Design review of the part built by this model. Coordinates are the model's own, in mm. Face numbers are marked on the shaded views. Coordinates: 2 decimals unless noted, no trailing zeros. Loops run counter-clockwise (first coordinate to the right, second up) from the corner with the lowest first, then second, coordinate; pieces in that order, holes last.
Q1. Add section B-B on y = -2.5. Give the boundary of the cut face in (x, z), and give its area (3 significant figures).
Q2. For P1, Ø1.5, axis at y = -1, z = -9.5, coming from the +X side; P2, Ø3, axis at x = 0, z = 14, coming from the -Y side; P3, Ø8, axis at x = -2, y = -7, coming from the -Z side; P4, Ø1.5, axis at y = -5.5, z = -4.5, coming from the +X side, all flat-tipped, find the tip position at first contact; note any pin that passes through.
Q3. Add section C-C on z = -6. Give the boundary of the cut face in (x, y).
Q4. Wall thickness on probe 1 along Z at (x, y) = (0, 2.7); probe 2 along X at (y, z) = (-3.2, 0); probe 3 along X at (y, z) = (-1.75, 1): over which ranges is each line inside the solid? List them lowest first.
Q5. Draft analysis for pull direction X (two halves, no side actions). For the marked faces 1 and 2, state which applies: released by +X, released by -X, zero draft, split by the parting line, or undercut.
Q6. Add section D-D on x = 7.5. Give the boundary of the cut face in (y, z).
Q7. Add section A-A on y = 3.75. Give the boundary of the cut face in (x, z).
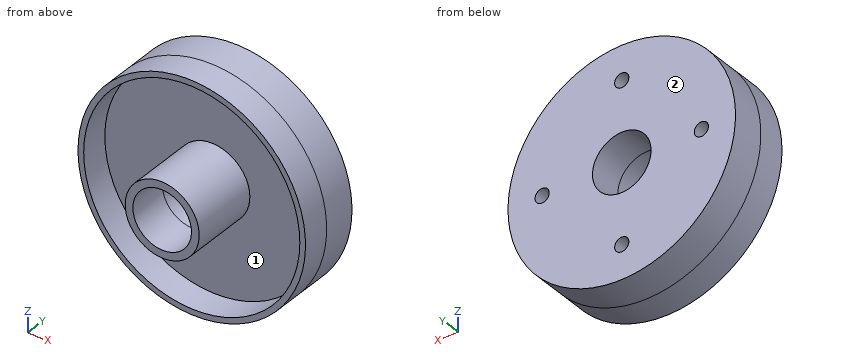
```python
from build123d import *

# Parameters (mm, degrees)
SKETCH_1_R             = 20
SKETCH_1_R_2           = 5.15
EXTRUDE_1_DEPTH        = 6
EXTRUDE_START          = 5
SKETCH_2_R             = 20
SKETCH_2_R_2           = 19
SKETCH_2_R_3           = 6.5
SKETCH_2_R_4           = 5.15
EXTRUDE_2_DEPTH        = 5
EXTRUDE_START_2        = 7
SKETCH_3_R             = 6.5
SKETCH_3_R_2           = 5.15
EXTRUDE_3_DEPTH        = 7
HOLE_WIZARD_M3_1_D     = 2.5
HOLE_WIZARD_M3_1_DEPTH = 5
HOLE_WIZARD_M3_1_TIP   = 0.751075774


with BuildPart() as part:
    # 草图1 → 凸台-拉伸1 (new body)
    with BuildSketch(Plane(origin=(0, 0, 0), x_dir=(1, 0, 0), z_dir=(0, 1, 0))):
        with Locations(Location((0, 0, 0), (0, 0, 270))):
            Circle(SKETCH_1_R)
        with Locations(Location((0, 0, 0), (0, 0, 270))):
            Circle(SKETCH_1_R_2, mode=Mode.SUBTRACT)
    extrude(amount=EXTRUDE_1_DEPTH)

    # 草图2 → 凸台-拉伸2 (add)
    # profile 1 of 2: a face of its own
    with BuildSketch(Plane.XZ.offset(EXTRUDE_START)):
        with Locations(Location((0, 0, 0), (0, 0, 270))):
            Circle(SKETCH_2_R)
        with Locations(Location((0, 0, 0), (0, 0, 270))):
            Circle(SKETCH_2_R_2, mode=Mode.SUBTRACT)
    # profile 2 of 2: a face of its own
    with BuildSketch(Plane.XZ.offset(EXTRUDE_START)):
        with Locations(Location((0, 0, 0), (0, 0, 90))):
            Circle(SKETCH_2_R_3)
        with Locations(Location((0, 0, 0), (0, 0, 270))):
            Circle(SKETCH_2_R_4, mode=Mode.SUBTRACT)
    extrude(amount=-EXTRUDE_2_DEPTH)

    # 草图3 → 凸台-拉伸3 (add)
    with BuildSketch(Plane.XZ.offset(5).offset(EXTRUDE_START_2)):
        with Locations(Location((0, 0, 0), (0, 0, 90))):
            Circle(SKETCH_3_R)
        with Locations(Location((0, 0, 0), (0, 0, 270))):
            Circle(SKETCH_3_R_2, mode=Mode.SUBTRACT)
    extrude(amount=-EXTRUDE_3_DEPTH)

    # M3 螺纹孔1
    with Locations(Plane(origin=(0, 6, 0), x_dir=(1, 0, 0), z_dir=(0, 1, 0))):
        with Locations((0, 14), (0, -14), (14, 0), (-14, 0)):
            Hole(HOLE_WIZARD_M3_1_D / 2, depth=HOLE_WIZARD_M3_1_DEPTH)
            with Locations((0, 0, -(HOLE_WIZARD_M3_1_DEPTH + HOLE_WIZARD_M3_1_TIP / 2))):  # 118° drill point
                Cone(0, HOLE_WIZARD_M3_1_D / 2, HOLE_WIZARD_M3_1_TIP, mode=Mode.SUBTRACT)


solid = part.part
```
Entries:
1. outline: circle Ø40 at (0, 0); circle Ø13 at (0, 0); hole circle Ø38 at (0, 0); hole circle Ø10.3 at (0, 0)
1. area: 172 mm2
2. P1: stops at x = 17.98
2. P2: stops at y = 0
2. P3: stops at z = -20
2. P4: stops at x = 19.61
3. outline: (-19.08, -5) - (-18.03, -5) - (-18.03, 0) - (-2.5, 0) - (-2.5, -12) - (2.5, -12) - (2.5, 0) - (18.03, 0) - (18.03, -5) - (19.08, -5) - (19.08, 6) - (-19.08, 6) - close
4. probe 1: z = -20 to -15.25, -12.75 to -5.15, 5.15 to 12.75, 15.25 to 20
4. probe 2: x = -20 to -19, -6.5 to -5.15, 5.15 to 6.5, 19 to 20
4. probe 3: x = -19.97 to -18.97, -6.42 to -5.05, 5.05 to 6.42, 18.97 to 19.97
5. face 1: undercut
5. face 2: zero draft
6. outline: (-5, -18.54) - (6, -18.54) - (6, 18.54) - (-5, 18.54) - (-5, 17.46) - (0, 17.46) - (0, -17.46) - (-5, -17.46) - close
7. outline: circle Ø40 at (0, 0); hole circle Ø2.5 at (-14, 0); hole circle Ø10.3 at (0, 0); hole circle Ø2.5 at (0, -14); hole circle Ø2.5 at (0, 14); hole circle Ø2.5 at (14, 0)
